The listing builds one solid part. Answer for the finished solid, in the listing's coordinates (mm). A direction names the side the tool comes from. Give positions to 0.01 mm unless a question says otherwise; leave off trailing zeros. Order: outer loops, then holes, each group sorted by start corner. A loop starts at its lowest first (then second) coordinate and runs counter-clockwise, first axis right, second up. Notation, with made-up numbers: (48.25, 11.25) - (82.25, 11.25) arc R16 cw to (82.25, 27.25) - close; hole circle Ø5 at (16, 5.25). An arc over 180 degrees is marked (long way). Answer as a JSON object with one key per item and string values. Group by question number.
Q1. Given pin 1 (3 mm diameter, centred on x = 48.5, z = -23, fed in from -Y); pin 2 (10 mm diameter, centred on x = 12.5, z = -59, fed in from -Y); pin 3 (5 mm diameter, centred on y = -6.5, z = -72, fed in from +X), each flat-ended and moving along its own axis, determine where each tip first touches the part or whether it passes through.
Q2. A cutting plane is placed at C-C, the plane z = -53.5. Give the vertices of the cut face in (x, y), and give its area (3 significant figures).
Q3. A cutting plane is placed at D-D, the plane x = 38.5. Give the vertices of the cut face in (y, z), and give its area (3 significant figures).
Q4. For faces 1 (the face through (33.662, -13, -73)), 2 (the face through (50.379, -13, -73)), 3 (the face through (77.58, 14, -38)), 4 (the face through (53.187, 27, -38)), determine the directions among +Z, -Z, +X, -X, +Y, -Y from which every point of the face is accessible in a straight line to the end or side of a thin tool.
Q5. A cutting plane is placed at A-A, the plane y = 7. Give the vertices of the cut face in (x, z), and give its area (3 significant figures).
Q6. Consider line 1 (Y direction, x = 27.5, z = -10.5); line 2 (X direction, y = 18.5, z = -67); line 3 (Y direction, x = 52.5, z = -12). Determine where each line is inside the solid, lowest interval first.
Q7. A cutting plane is placed at B-B, the plane x = 69. Give the vertices of the cut face in (y, z), and give its area (3 significant figures).
from build123d import *

# Parameters (mm, degrees)
SKETCH1_W           = 84.040425815
SKETCH1_H           = 30.284008864
BOSS_EXTRUDE1_DEPTH = 76.2
CUT_EXTRUDE1_DEPTH  = 118.415307197
SKETCH3_W           = 16.716926531
SKETCH3_H           = 25.4
BOSS_EXTRUDE2_DEPTH = 6.35
SKETCH4_R           = 8.358463265
BOSS_EXTRUDE3_DEPTH = 76.2


with BuildPart() as part:
    # Sketch1 → Boss-Extrude1 (new body)
    with BuildSketch(Plane.XY):
        with Locations((42.020212908, 15.142004432)):
            Rectangle(SKETCH1_W, SKETCH1_H)
    extrude(amount=-BOSS_EXTRUDE1_DEPTH)

    # Sketch2 → Cut-Extrude1 (cut, through all)
    with BuildSketch(Plane.XY):
        Polygon((30.853035266, 30.284008864), (53.187390549, 30.284008864), (53.187390549, 22.664008864), (77.580212908, 22.664008864), (77.580212908, 4.884008864), (6.460212908, 4.884008864), (6.460212908, 22.664008864), (30.853035266, 22.664008864), align=None)
    extrude(amount=-CUT_EXTRUDE1_DEPTH, mode=Mode.SUBTRACT)

    # Sketch3 → Boss-Extrude2 (add)
    with BuildSketch(Plane.XY.offset(-76.2)):
        with Locations((42.020212908, -12.7)):
            Rectangle(SKETCH3_W, SKETCH3_H)
    extrude(amount=BOSS_EXTRUDE2_DEPTH)

    # Sketch4 → Boss-Extrude3 (add)
    with BuildSketch(Plane.XY.offset(-76.2)):
        with Locations((42.020212908, -25.4)):
            Circle(SKETCH4_R)
    extrude(amount=BOSS_EXTRUDE3_DEPTH)


solid = part.part
Reply:
{
 "1": {"pin 1": "stops at y = -32.11", "pin 2": "stops at y = 0", "pin 3": "stops at x = 50.38"},
 "2": {"outline": "(0, 0) - (84.04, 0) - (84.04, 30.28) - (53.19, 30.28) - (53.19, 22.66) - (77.58, 22.66) - (77.58, 4.88) - (6.46, 4.88) - (6.46, 22.66) - (30.85, 22.66) - (30.85, 30.28) - (0, 30.28) - close; circle Ø16.72 at (42.02, -25.4)", "area": "1,330 mm^2"},
 "3": {"outline": "(-32.98, -76.2) - (4.88, -76.2) - (4.88, 0) - (0, 0) - (0, -69.85) - (-17.82, -69.85) - (-17.82, 0) - (-32.98, 0) - close", "area": "1,640 mm^2"},
 "4": {"face 1": "+Z, -Z, -X, -Y", "face 2": "+Z, -Z, +X, -Y", "face 3": "+Z, -Z", "face 4": "+Z, -Z, +Y"},
 "5": {"outline": "(0, -76.2) - (6.46, -76.2) - (6.46, 0) - (0, 0) - close; (77.58, -76.2) - (84.04, -76.2) - (84.04, 0) - (77.58, 0) - close", "area": "985 mm^2"},
 "6": {"line 1": "y = 0 to 4.88, 22.66 to 30.28", "line 2": "x = 0 to 6.46, 77.58 to 84.04", "line 3": "y = 0 to 4.88"},
 "7": {"outline": "(0, -76.2) - (4.88, -76.2) - (4.88, 0) - (0, 0) - close; (22.66, -76.2) - (30.28, -76.2) - (30.28, 0) - (22.66, 0) - close", "area": "953 mm^2"}
}
